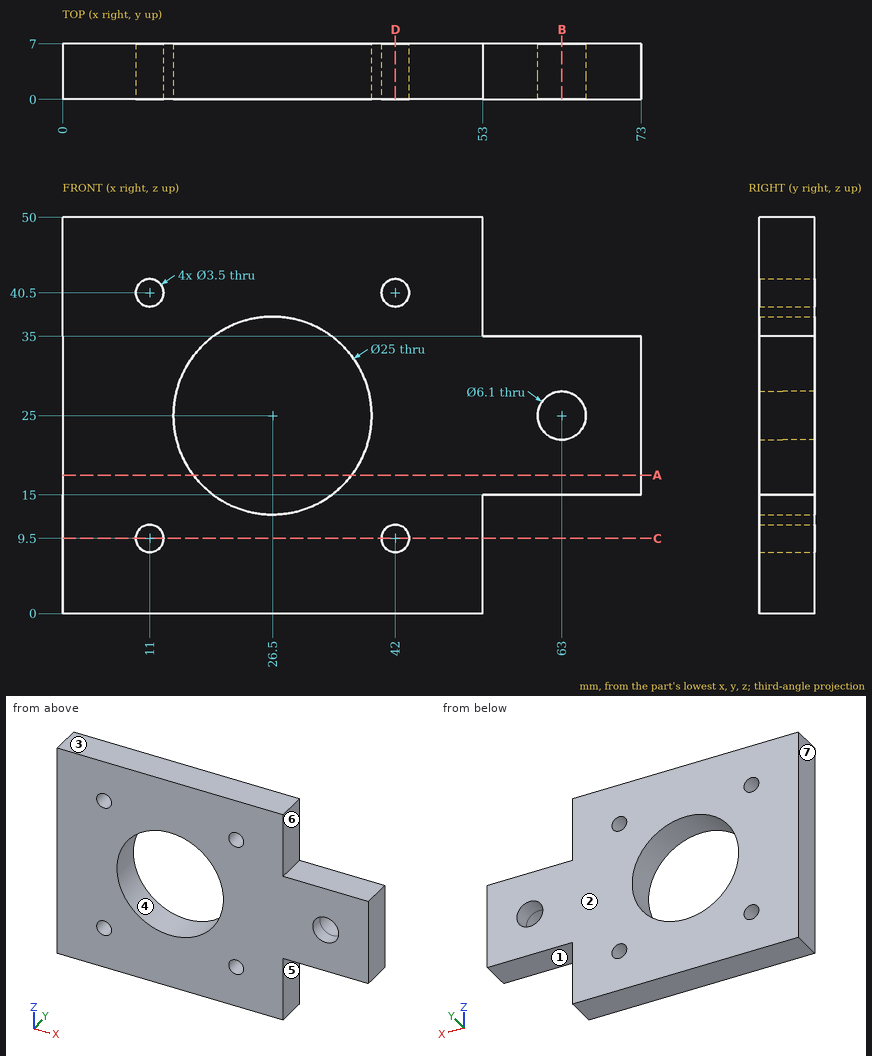
Can you work these out from the drawing? Everything is in mm from the part's minimum corner. A direction names the side the tool comes from. Coordinates: 2 decimals unless noted, no trailing zeros. Loops run counter-clockwise (first coordinate to the right, second up) from the corner with the lowest first, then second, coordinate; pieces in that order, holes last.
1. For P1, Ø2, axis at x = 62.5, y = 3, coming from the -Z side; P2, Ø2, axis at x = 42, z = 40.5, coming from the +Y side; P3, Ø2, axis at y = 4.5, z = 44.5, coming from the +X side, each with a flat end and sliding along its axis, tell me the tip position at first contact or that it passes through.
2. Imagine slicing it at B-B, the plane x = 63. Please give me the cut outline in (y, z).
3. If we mould it in two halves opening along Z, with no side actions, what happens to the marked faces 1, 2, 3 and 4? For each: pulls with the +Z half, pulls with the -Z half, needs draft (parallel to the pull), parting line crosses it, or undercut.
4. I need wall thicknesses on L1, parallel to Z at x = 42, y = 2; L2, parallel to X at y = 2, z = 9.5; L3, parallel to X at y = 5.1, z = 25. Which ranges of each line are inside material? Lowest first, please.
5. Imagine slicing it at D-D, the plane x = 42. Please give me the cut outline in (y, z).
6. Imagine slicing it at A-A, the plane z = 17.5. Please give me the cut outline in (x, y).
7. For the marked faces 5, 6 and 7, which set-ups out of +Z, -Z, +X, -X, +Y, -Y let a thin tool reach every point of the face, with its end or its side?
8. Imagine slicing it at C-C, the plane z = 9.5. Please give me the cut outline in (x, y).
Taken from the geometry:
1. P1: stops at z = 15
1. P2: passes through
1. P3: stops at x = 53
2. outline: (0, 15) - (7, 15) - (7, 21.95) - (0, 21.95) - close; (0, 28.05) - (7, 28.05) - (7, 35) - (0, 35) - close
3. face 1: pulls with the -Z half
3. face 2: needs draft
3. face 3: pulls with the +Z half
3. face 4: undercut
4. L1: z = 0 to 7.75, 11.25 to 38.75, 42.25 to 50
4. L2: x = 0 to 9.25, 12.75 to 40.25, 43.75 to 53
4. L3: x = 0 to 14, 39 to 59.95, 66.05 to 73
5. outline: (0, 0) - (7, 0) - (7, 7.75) - (0, 7.75) - close; (0, 11.25) - (7, 11.25) - (7, 38.75) - (0, 38.75) - close; (0, 42.25) - (7, 42.25) - (7, 50) - (0, 50) - close
6. outline: (0, 0) - (16.5, 0) - (16.5, 7) - (0, 7) - close; (36.5, 0) - (73, 0) - (73, 7) - (36.5, 7) - close
7. face 5: -Z, +X, +Y, -Y
7. face 6: +Z, +X, +Y, -Y
7. face 7: +Z, -Z, -X, +Y, -Y
8. outline: (0, 0) - (9.25, 0) - (9.25, 7) - (0, 7) - close; (12.75, 0) - (40.25, 0) - (40.25, 7) - (12.75, 7) - close; (43.75, 0) - (53, 0) - (53, 7) - (43.75, 7) - close
